from build123d import *

# Parameters (mm, degrees)
PAD_DEPTH               = 3
PAD001_DEPTH            = 2
PAD002_DEPTH            = 20
PAD003_DEPTH            = 2.5
PAD_MIRRORED_2_DEPTH    = 3
PAD001_MIRRORED_2_DEPTH = 2
PAD002_MIRRORED_2_DEPTH = 20
PAD003_MIRRORED_2_DEPTH = 2.5
CHAMFER_SIZE2           = 1
CHAMFER_SIZE            = 3


with BuildPart() as part:
    # Sketch → Pad (new body)
    with BuildSketch(Plane.XY):
        Polygon((0, 4.25), (1, 4.25), (1, 3), (3, 3), (3, 0), (0, 0), align=None)
    pad = extrude(amount=PAD_DEPTH)

    # Sketch001 (on Face8 of Pad) → Pad001 (join)
    with BuildSketch(Plane.XY.offset(3)):
        with BuildLine():
            ThreePointArc((10.85, 0), (7.672109, 7.672109), (0, 10.85))
            Line((0, 10.85), (0, 0))
            Line((0, 0), (10.85, 0))
        make_face()
    pad001 = extrude(amount=PAD001_DEPTH)

    # Sketch002 (on Face12 of Pad001) → Pad002 (join)
    with BuildSketch(Plane.XY.offset(5)):
        with BuildLine():
            ThreePointArc((10.85, 0), (7.672109, 7.672109), (0, 10.85))
            Line((0, 0), (0, 10.85))
            Line((0, 0), (10.85, 0))
        make_face()
    pad002 = extrude(amount=PAD002_DEPTH)

    # Sketch003 (on Face5 of Pad002) → Pad003 (join)
    with BuildSketch(Plane(origin=(0, 0, 3), x_dir=(1, 0, 0), z_dir=(0, 0, -1))):
        with BuildLine():
            ThreePointArc((1.25, -5.868347), (2.641923, -5.387044), (3.874663, -4.581156))
            Line((3.874663, -4.581156), (8.072214, -9.544074))
            ThreePointArc((0, -12.5), (4.298201, -11.737779), (8.072214, -9.544074))
            Line((0, -8.868347), (0, -12.5))
            Line((1.25, -8.868347), (0, -8.868347))
            Line((1.25, -8.868347), (1.25, -5.868347))
        make_face()
    pad003 = extrude(amount=PAD003_DEPTH)

    # Sketch Mirrored 2 → Pad Mirrored 2 (add)
    with BuildSketch(Plane(origin=(0, 0, 0), x_dir=(-1, 0, 0), z_dir=(0, 0, -1))):
        Polygon((0, 4.25), (1, 4.25), (1, 3), (3, 3), (3, 0), (0, 0), align=None)
    pad_mirrored_2 = extrude(amount=-PAD_MIRRORED_2_DEPTH)

    # Sketch001 Mirrored 2 → Pad001 Mirrored 2 (add)
    with BuildSketch(Plane(origin=(0, 0, 3), x_dir=(-1, 0, 0), z_dir=(0, 0, -1))):
        with BuildLine():
            ThreePointArc((10.85, 0), (7.672109, 7.672109), (0, 10.85))
            Line((0, 10.85), (0, 0))
            Line((0, 0), (10.85, 0))
        make_face()
    pad001_mirrored_2 = extrude(amount=-PAD001_MIRRORED_2_DEPTH)

    # Sketch002 Mirrored 2 → Pad002 Mirrored 2 (add)
    with BuildSketch(Plane(origin=(0, 0, 5), x_dir=(-1, 0, 0), z_dir=(0, 0, -1))):
        with BuildLine():
            ThreePointArc((10.85, 0), (7.672109, 7.672109), (0, 10.85))
            Line((0, 0), (0, 10.85))
            Line((0, 0), (10.85, 0))
        make_face()
    pad002_mirrored_2 = extrude(amount=-PAD002_MIRRORED_2_DEPTH)

    # Sketch003 Mirrored 2 → Pad003 Mirrored 2 (add)
    with BuildSketch(Plane(origin=(0, 0, 3), x_dir=(-1, 0, 0), z_dir=(0, 0, 1))):
        with BuildLine():
            ThreePointArc((1.25, -5.868347), (2.641923, -5.387044), (3.874663, -4.581156))
            Line((3.874663, -4.581156), (8.072214, -9.544074))
            ThreePointArc((0, -12.5), (4.298201, -11.737779), (8.072214, -9.544074))
            Line((0, -8.868347), (0, -12.5))
            Line((1.25, -8.868347), (0, -8.868347))
            Line((1.25, -8.868347), (1.25, -5.868347))
        make_face()
    pad003_mirrored_2 = extrude(amount=-PAD003_MIRRORED_2_DEPTH)

    # Mirrored001: Pad, Pad001, Pad002, Pad003, Pad Mirrored 2, Pad001 Mirrored 2, Pad002 Mirrored 2, Pad003 Mirrored 2 across Sketch H_Axis
    add(pad.mirror(Plane.ZX))
    add(pad001.mirror(Plane.ZX))
    add(pad002.mirror(Plane.ZX))
    add(pad003.mirror(Plane.ZX))
    add(pad_mirrored_2.mirror(Plane.ZX))
    add(pad001_mirrored_2.mirror(Plane.ZX))
    add(pad002_mirrored_2.mirror(Plane.ZX))
    add(pad003_mirrored_2.mirror(Plane.ZX))

    # Chamfer
    chamfer_edges = [part.edges().sort_by_distance(p)[0] for p in [
        (-7.672109, -7.672109, 25),
    ]]
    chamfer_side = part.faces().sort_by_distance((-7.672109, -7.672109, 15))[0]
    chamfer(chamfer_edges, length=CHAMFER_SIZE, length2=CHAMFER_SIZE2, reference=chamfer_side)


solid = part.part
The listing builds one solid part. Answer for the finished solid, in the listing's coordinates (mm). A direction names the side the tool comes from. Round coordinates to 2 decimals unless told otherwise and drop trailing zeros. Loops run counter-clockwise (first coordinate to the right, second up) from the corner with the lowest first, then second, coordinate; pieces in that order, holes last. Notation, with made-up numbers: M -36,-28 L -28,-28 A8 cw -28,-17 Z; hole C 2.5,41 d11. An arc over 180 degrees is marked long. Return JSON: item names as keys, results as strings.
Q1. Which of the six approach directions +Z, -Z, +X, -X, +Y, -Y give full straight-line access (tool end or side, diameter ignored) to faces 1 (the face through (1, 4, 1)), 2 (the face through (-3, 0, 1)), 3 (the face through (0, 4.25, 1)), 4 (the face through (1.25, -7, 2))?
Results list:
{"face 1": "-Z, +X", "face 2": "-Z, -X", "face 3": "-Z, +X, -X", "face 4": "-Z"}
Q2. The mould has two halves that part along Y. Classify faces 5 (the face through (5.944, -7.028, 1.768)), 6 (the face through (-0.1, -11.3, 3)): released by +Y, released by -Y, zero draft, split by the parting line, or undercut.
Results list:
{"face 5": "undercut", "face 6": "zero draft"}
Q3. Each of these flat-tipped pins is pushed along its axis until it touches: pin 1 Ø5 at (y, z) = (-8, 5) entering from +X; pin 2 Ø2 at (x, z) = (-2, 1.5) entering from +Y; pin 3 Ø1.2 at (y, z) = (7.5, 2) entering from -X; pin 4 Ø10 at (x, y) = (6, -9.5) entering from +Z. Where does it stop, or does it pass through?
Results list:
{"pin 1": "stops at x = 9.35", "pin 2": "stops at y = 12.46", "pin 3": "stops at x = -6.85", "pin 4": "stops at z = 25"}
Q4. Find section A-A, the plane z = 5.5. Determine the outline of the cut face in (x, y).
Results list:
{"outline": "M -10.85,0 A10.85 ccw 0,-10.85 A10.85 ccw 10.85,0 A10.85 ccw 0,10.85 A10.85 ccw Z"}
Q5. Find section B-B, the plane z = 23. Determine the outline of the cut face in (x, y), plus the area to 3 significant figures.
Results list:
{"outline": "M -10.52,0 A10.52 ccw 0,-10.52 A10.52 ccw 10.52,0 A10.52 ccw 0,10.52 A10.52 ccw Z", "area": "347 mm2"}
Q6. Find the intervals of material crossed by line 1 along Z through (x, y) = (-6.5, 2.5); line 2 along Y through (x, z) = (-0.25, 20.25); line 3 along Y through (x, z) = (-6.25, 14), in increasing order. Write a range as from..to.
Results list:
{"line 1": "z = 3..25", "line 2": "y = -10.85..10.85", "line 3": "y = -8.87..8.87"}
